Could you check a few things on this model? Use its own coordinates, in mm. A direction names the side the tool comes from. Coordinates: 2 decimals unless noted, no trailing zeros. Order: outer loops, then holes, each group sorted by start corner. A loop starts at its lowest first (then second) coordinate and runs counter-clockwise, first axis right, second up.
```python
from build123d import *

# Parameters (mm, degrees)
SKETCH003_R     = 2.5
SKETCH003_R_2   = 1.3
PAD003_DEPTH    = 6
SKETCH004_R     = 1.3
PAD004_DEPTH    = 5
CHAMFER001_SIZE = 0.2


with BuildPart() as part:
    # Sketch003 → Pad003 (new body)
    with BuildSketch(Plane.XY):
        Circle(SKETCH003_R)
        Circle(SKETCH003_R_2, mode=Mode.SUBTRACT)
    extrude(amount=PAD003_DEPTH)

    # Sketch004 → Pad004 (join)
    with BuildSketch(Plane.XY.offset(0.5)):
        Polygon((2.53, -1.460696), (2.53, 1.460696), (0, 2.921392), (-2.53, 1.460696), (-2.53, -1.460696), (0, -2.921392), align=None)
        Circle(SKETCH004_R, mode=Mode.SUBTRACT)
    extrude(amount=PAD004_DEPTH)

    # Chamfer001
    chamfer001_edges = [part.edges().sort_by_distance(p)[0] for p in [
        (-2.5, 0, 6),
        (-2.5, 0, 0),
    ]]
    chamfer(chamfer001_edges, length=CHAMFER001_SIZE)


with BuildPart() as part_1:
    # Body002 placement: moved
    add(part.part.moved(Location((49.5, 0, 0))))


solid = part_1.part
```
Item 1: Suppose I cut it at B-B (z = 2.9). List the corners of the cut face in (x, y) for me.
Item 2: For pin 1 Ø1 at (y, z) = (-2, 1.5) entering from +X, with a flat end and sliding along its axis, tell me the tip position at first contact or that it passes through.
Item 3: Which directions (+Z, -Z, +X, -X, +Y, -Y) give clear straight access to the entire face, cutting with the end or side of a thin tool? Please do faces 1 (the face through (51.81, -0.96, 0.35)), 2 (the face through (51, 0, 0)).
Item 4: Thinking about a two-plate mould opening in X: for faces 3 (the face through (51.81, -0.96, 5.65)), 4 (the face through (48.2, 0.06, 2.96)), 5 (the face through (51, 0, 6)), which applies, +X half, -X half, draft (parallel to the pull), parting line (faces both ways), or undercut?
Item 5: I need wall thicknesses on line 1 (X direction, y = 0.65, z = 1.5); line 2 (X direction, y = -0.45, z = 2.2); line 3 (Z direction, x = 51.5, y = -1.7). Which ranges of each line are inside material? Lowest first, please.
Geometry results:
1. outline: (46.97, -1.46) - (49.5, -2.92) - (52.03, -1.46) - (52.03, 1.46) - (49.5, 2.92) - (46.97, 1.46) - close; hole circle Ø2.6 at (49.5, 0)
2. pin 1: stops at x = 51.96
3. face 1: -Z
3. face 2: -Z, +X, -X, +Y, -Y
4. face 3: parting line
4. face 4: undercut
4. face 5: draft
5. line 1: x = 46.97 to 48.37, 50.63 to 52.03
5. line 2: x = 46.97 to 48.28, 50.72 to 52.03
5. line 3: z = 0.5 to 5.5
